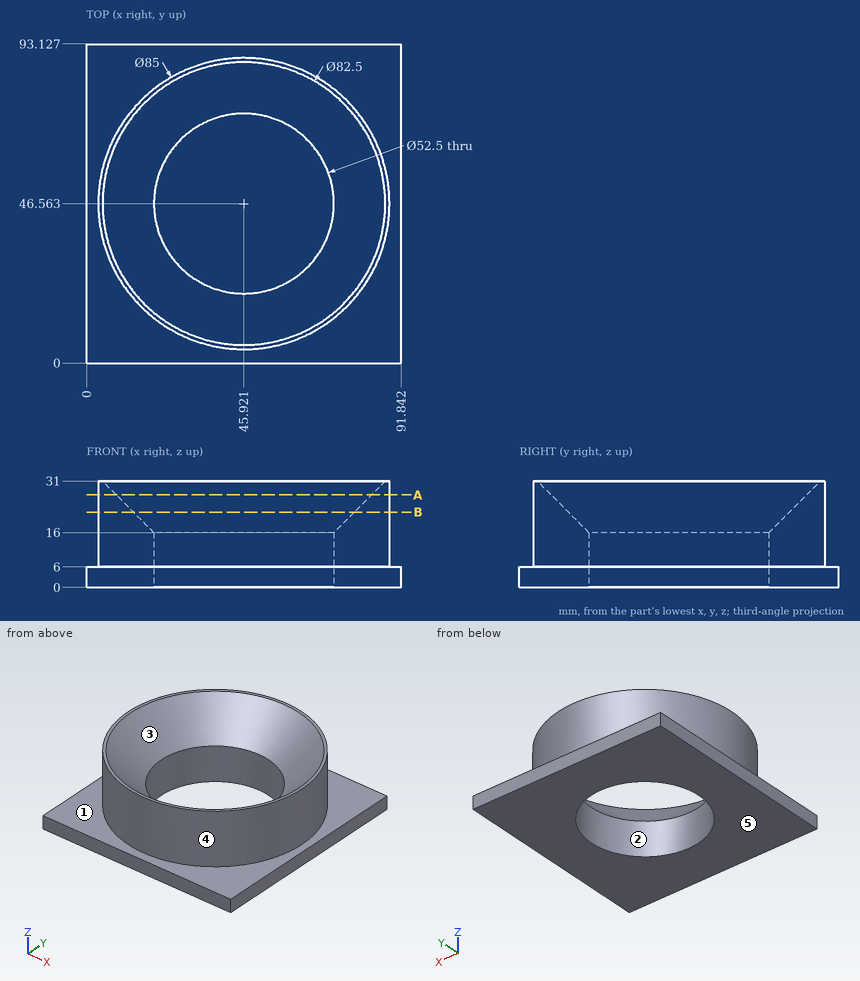
For this review, use the dimensioned drawing (mm, ordinates from the lowest corner) and the shaded views. A direction names the side the tool comes from. Coordinates: 2 decimals unless noted, no trailing zeros. Loops run counter-clockwise (first coordinate to the right, second up) from the corner with the lowest first, then second, coordinate; pieces in that order, holes last. Notation, with made-up numbers: (25, 68) -> (63, 68) arc R19 cw to (63, 99) -> close; hole circle Ø6 at (70, 44). An arc over 180 degrees is marked (long way). Return JSON: item names as keys, results as strings. Group by question number.
(1) For pin 1 Ø3 at (y, z) = (24.5, 9.5) entering from +X (1 decimal); pin 2 Ø2 at (y, z) = (73, 25.5) entering from +X; pin 3 Ø3 at (y, z) = (68, 13) entering from +X (1 decimal), all flat-tipped, find the tip position at first contact; note any pin that passes through.
(2) Consider section A-A, the plane z = 27. Give the boundary of the cut face in (x, y).
(3) Tool access review of the marked faces 1 and 2: name each direction out of +Z, -Z, +X, -X, +Y, -Y from which nothing blocks a thin tool from reaching the whole face with its end or side.
(4) Mouldability with a two-part tool opening along X and no side actions: class the marked faces 3, 4 and 5 as pulls with the +X half, pulls with the -X half, needs draft (parallel to the pull), parting line crosses it, or undercut.
(5) Consider section B-B, the plane z = 22. Give the boundary of the cut face in (x, y).
(6) To check wall thickness, follow L1, parallel to Z at x = 72.5, y = 86; L2, parallel to X at y = 52, z = 28; L3, parallel to Y at x = 16, z = 29.5 (1 decimal). State the ranges of each line that lie inside material, in increasing order.
Results below:
{
 "1": {"pin 1": "stops at x = 83.1", "pin 2": "stops at x = 79.97", "pin 3": "stops at x = 83.5"},
 "2": {"outline": "circle Ø85 at (45.92, 46.56); hole circle Ø74.5 at (45.92, 46.56)"},
 "3": {"face 1": "+Z", "face 2": "+Z, -Z"},
 "4": {"face 3": "undercut", "face 4": "parting line crosses it", "face 5": "needs draft"},
 "5": {"outline": "circle Ø85 at (45.92, 46.56); hole circle Ø64.5 at (45.92, 46.56)"},
 "6": {"L1": "z = 0 to 6", "L2": "x = 3.77 to 8.06, 83.78 to 88.07", "L3": "y = 16.4 to 20.4, 72.7 to 76.7"}
}
